Verification items for this drawing (mm, ordinates from the low corner). Give positions to 0.01 mm unless a question says otherwise; leave off trailing zeros. Loops run counter-clockwise (first coordinate to the right, second up) from the corner with the lowest first, then second, coordinate; pieces in that order, holes last. Notation, with made-up numbers: (-27, -27) -> (23, -27) arc R22 cw to (23, 1) -> close; hole circle Ø10 at (-1, 36). An arc over 180 degrees is marked (long way). Write each question's results on one line, items separated by ' | '. Start each with the question number.
Item 1: Cross-section at C-C on y = 446. Enter the section's corners in (x, z), then the cut area to 3 significant figures.
Item 2: Gauge pin test, flat ends, axial feed: pin 1 Ø14.5 at (x, y) = (13.5, 305) entering from -Z; pin 2 Ø15 at (x, z) = (17.5, 111) entering from -Y; pin 3 Ø5 at (x, z) = (26.5, 119.5) entering from +Y. Record the tip position at first contact, or that the pin passes through.
Item 3: Cross-section at A-A on x = 28.5. Enter the section's corners in (y, z).
Item 4: Scan lines: line 1 along Y through (x, z) = (22, 23); line 2 along Z through (x, y) = (45, 74). Record each from-to range of solid material in increasing order.
Item 5: Cross-section at B-B on z = 23. Enter the section's corners in (x, y).
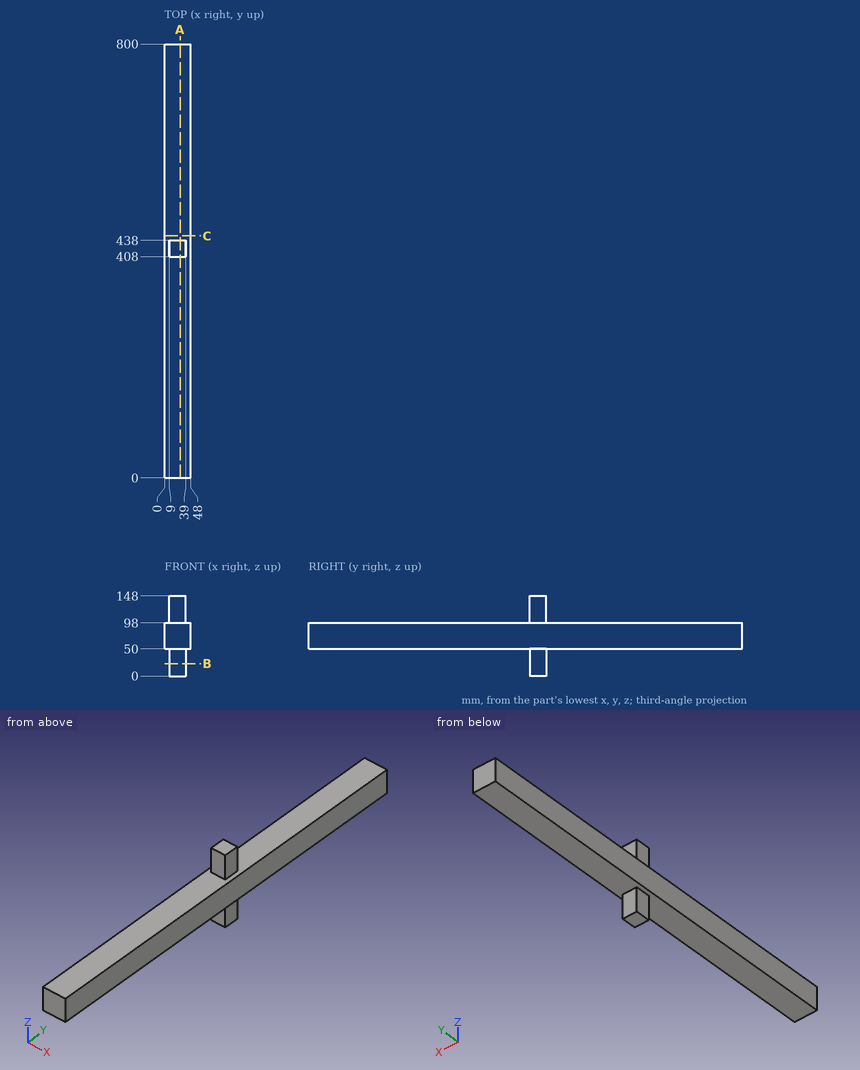
Answer sheet:
1) outline: (0, 50) -> (48, 50) -> (48, 98) -> (0, 98) -> close | area: 2,300 mm²
2) pin 1: stops at z = 50 | pin 2: stops at y = 408 | pin 3: stops at y = 438
3) outline: (0, 50) -> (408, 50) -> (408, 0) -> (438, 0) -> (438, 50) -> (800, 50) -> (800, 98) -> (438, 98) -> (438, 148) -> (408, 148) -> (408, 98) -> (0, 98) -> close
4) line 1: y = 408 to 438 | line 2: z = 50 to 98
5) outline: (9, 408) -> (39, 408) -> (39, 438) -> (9, 438) -> close
